from build123d import *

# Parameters (mm, degrees)
SKETCH1_R           = 1.6
BOSS_EXTRUDE1_DEPTH = 1.5
FILLET1_R           = 0.2


with BuildPart() as part:
    # Sketch1 → Boss-Extrude1 (new body)
    with BuildSketch(Plane.XY):
        with BuildLine():
            Line((-3, 0), (-3, -31.38))
            ThreePointArc((-3, -31.38), (0, -34.38), (3, -31.38))
            Line((3, -31.38), (3, 0))
            ThreePointArc((3, 0), (0, 3), (-3, 0))
        make_face()
        Circle(SKETCH1_R, mode=Mode.SUBTRACT)
        with Locations((0, -31.38)):
            Circle(SKETCH1_R, mode=Mode.SUBTRACT)
    extrude(amount=BOSS_EXTRUDE1_DEPTH)

    # Fillet1
    fillet1_edges = [part.edges().sort_by_distance(p)[0] for p in [
        (0, -34.38, 1.5),
        (3, -15.69, 1.5),
        (0, 3, 1.5),
        (3, -15.69, 0),
        (0, -34.38, 0),
        (-3, -15.69, 0),
        (0, 3, 0),
        (-3, -15.69, 1.5),
    ]]
    fillet(fillet1_edges, radius=FILLET1_R)


solid = part.part
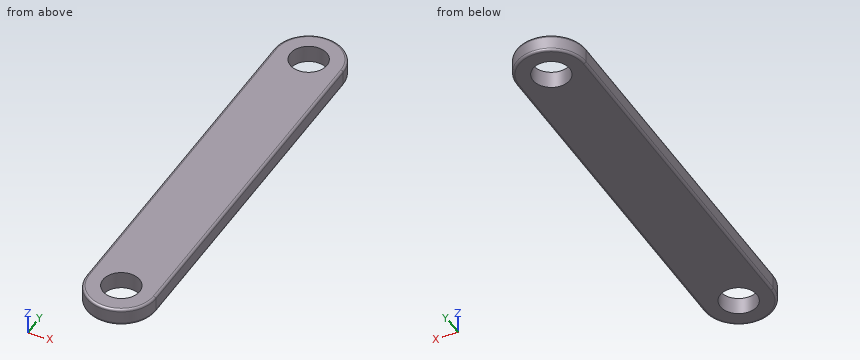
Design review of the part built by this model. Coordinates are the model's own, in mm. Coordinates: 2 decimals unless noted, no trailing zeros. Order: outer loops, then holes, each group sorted by start corner. A loop starts at its lowest first (then second) coordinate and runs counter-clockwise, first axis right, second up. Notation, with made-up numbers: M 3.5,60.25 L 27.5,60.25 A12 ccw 27.5,79.25 Z; hole C 75,86 d1. An arc over 180 degrees is marked long. Use a Markdown table: item, result.
(1) Wall thickness on probe 1 along Y at (x, z) = (-0.1, 1.35); probe 2 along Y at (x, z) = (0.35, 1.15); probe 3 along Y at (x, z) = (-2.3, 1.1): over which ranges is each line inside the solid? List them lowest first.
Worked answers:
| item | result |
|---|---|
| probe 1 | y = -34.37 to -32.98, -29.78 to -1.6, 1.6 to 2.99 |
| probe 2 | y = -34.36 to -32.94, -29.82 to -1.56, 1.56 to 2.98 |
| probe 3 | y = -33.31 to 1.93 |
(2) Add section A-A (x = 0). Give the boundary of the cut face in (y, z).
Worked answers:
| item | result |
|---|---|
| outline | M -34.38,0.2 A0.2 ccw -34.18,0 L -32.98,0 L -32.98,1.5 L -34.18,1.5 A0.2 ccw -34.38,1.3 Z; M -29.78,0 L -1.6,0 L -1.6,1.5 L -29.78,1.5 Z; M 1.6,0 L 2.8,0 A0.2 ccw 3,0.2 L 3,1.3 A0.2 ccw 2.8,1.5 L 1.6,1.5 Z |
(3) For P1, Ø3, axis at x = 0, y = 0, coming from the -Z side, flat-tipped, find the tip position at first contact; note if it passes through.
Worked answers:
| item | result |
|---|---|
| P1 | passes through |
(4) Add section B-B (z = 0.75). Give the boundary of the cut face in (x, y).
Worked answers:
| item | result |
|---|---|
| outline | M -3,-31.38 A3 ccw 3,-31.38 L 3,0 A3 ccw -3,0 Z; hole C 0,-31.38 d3.2; hole C 0,0 d3.2 |
